Design review of the part built by this model. Coordinates are the model's own, in mm. A direction names the side the tool comes from. Give positions to 0.01 mm unless a question says otherwise; leave off trailing zeros. Loops run counter-clockwise (first coordinate to the right, second up) from the corner with the lowest first, then second, coordinate; pieces in that order, holes last. Notation, with made-up numbers: (54.5, 86) -> (113.5, 86) arc R35 cw to (113.5, 118) -> close; hole circle Ø6 at (1, -16). An arc over 180 degrees is marked (long way). Use CSV: the item, a comma, the result in double quotes. Start each with the question number.
Item 1: Wall thickness on line 1 along Y through (x, z) = (53, 1.6); line 2 along X through (y, z) = (-12, 0.4); line 3 along Y through (x, z) = (-33, 2.55): over which ranges is each line inside the solid? List them lowest first. Write a range as from..to.
Item 2: We need section A-A (x = -23). State the section outline as (y, z) points, plus the area to 3 significant figures.
Item 3: For faces 1 (the face through (1, -49, 1)), 2 (the face through (-60, 1, 1)), list the 3-axis set-ups (+Z, -Z, +X, -X, +Y, -Y) from which the entire face can be reached by the end or side of a thin tool; tool diameter is ignored.
Item 4: Clearance check with a flat-ended pin moving along its axis: pin 1 (6 mm diameter, centred on x = -36, y = -29.5, fed in from -Z). State where the tip first meets the part, or that it passes through.
Item 5: We need section B-B (y = 37). State the section outline as (x, z) points.
Item 6: The part is to be moulded in two halves that separate along X. For faces 3 (the face through (-41, 1, 0)), 4 (the face through (58.196, -67.289, 1.521)), 5 (the face through (-58.289, -67.196, 1.521)), 6 (the face through (50, -62, 2)), say which applies: +X half, -X half, draft (parallel to the pull), parting line (faces both ways), or undercut.
Item 7: We need section C-C (z = 0.6). State the section outline as (x, y) points, plus the area to 3 significant figures.
Autodesk Inventor part; units mm, degrees
ref_plane "YZ Plane" through (0, 0, 0) normal (1, 0, 0) x (0, 1, 0)
ref_plane "XZ Plane" through (0, 0, 0) normal (0, 1, 0) x (-1, 0, 0)
ref_plane "XY Plane" through (0, 0, 0) normal (0, 0, 1) x (1, 0, 0)
sketch "Sketch1" plane through (0, 0, 0) normal (0, 0, 1) x (1, 0, 0)
  line L0 (-60, -69) -> (60, -69)
  line L1 (60, -69) -> (60, 69)
  line L2 (60, 69) -> (-60, 69)
  line L3 (-60, 69) -> (-60, -69)
  line L4 (-60, -69) -> (60, 69) construction
  line L5 (60, -69) -> (-60, 69) construction
  line L6 (40, -49) -> (-40, -49)
  line L7 (-40, -49) -> (-40, 49)
  line L8 (-40, 49) -> (40, 49)
  line L9 (40, 49) -> (40, -49)
  line L10 (40, -49) -> (-40, 49) construction
  line L11 (-40, -49) -> (40, 49) construction
  point P0 (0, 0)
  dimension "d172" = 80
  dimension "d180" = 20
  dimension "d181" = 20
  dimension "d182" = 98
extrude "Plate5" add sketch "Sketch1" along normal blind 3
sketch "Sketch9" plane through (0, 0, 3) normal (0, 0, 1) x (1, 0, 0)
  circle A0 centre (53, -62) radius 3
  line L0 (53, 62) -> (-53, 62) construction
  line L1 (-53, 62) -> (-53, -62) construction
  line L2 (-53, -62) -> (53, -62) construction
  line L3 (53, -62) -> (53, 62) construction
  line L4 (53, 62) -> (-53, -62) construction
  line L5 (-53, 62) -> (53, -62) construction
  circle A1 centre (-53, -62) radius 3
  circle A2 centre (53, 62) radius 3
  circle A3 centre (-53, 62) radius 3
  line L6 (-40, -49) -> (-40, 49)
  line L7 (-40, 49) -> (40, 49)
  line L8 (40, 49) -> (40, -49)
  line L9 (40, -49) -> (-40, -49)
  line L10 (60, -69) -> (-60, -69)
  line L11 (60, 69) -> (60, -69)
  line L12 (-60, 69) -> (60, 69)
  line L13 (-60, -69) -> (-60, 69)
  circle A4 centre (-53, 0) radius 3 construction
  circle A5 centre (53, 0) radius 3 construction
  point P0 (0, 0)
  dimension "d174" = 6
  dimension "d183" = 7
  dimension "d184" = 7
extrude "Cut2" cut sketch "Sketch9" against normal blind 3 contours A0 | A1 | A2 | A3
fillet "Corner Round1" radius 6 4 edges at (60, 69, 1.5) (-60, 69, 1.5) (-60, -69, 1.5) (60, -69, 1.5)
properties part number "ANP 1421 FDS Diam way flange 1" material "Stainless Steel"
Results found:
1,line 1,"-69..-65, -59..59, 65..69"
1,line 2,"-60..-40, 40..60"
1,line 3,"-69..-49, 49..69"
2,outline,"(-69, 0) -> (-49, 0) -> (-49, 3) -> (-69, 3) -> close; (49, 0) -> (69, 0) -> (69, 3) -> (49, 3) -> close"
2,area,"120 mm²"
3,face 1,"+Z, -Z"
3,face 2,"+Z, -Z, -X, +Y, -Y"
4,pin 1,"through"
5,outline,"(-60, 0) -> (-40, 0) -> (-40, 3) -> (-60, 3) -> close; (40, 0) -> (60, 0) -> (60, 3) -> (40, 3) -> close"
6,face 3,"draft"
6,face 4,"+X half"
6,face 5,"-X half"
6,face 6,"undercut"
7,outline,"(-60, -63) arc R6 ccw to (-54, -69) -> (54, -69) arc R6 ccw to (60, -63) -> (60, 63) arc R6 ccw to (54, 69) -> (-54, 69) arc R6 ccw to (-60, 63) -> close; hole circle Ø6 at (-53, -62); hole circle Ø6 at (-53, 62); hole (-40, -49) -> (40, -49) -> (40, 49) -> (-40, 49) -> close; hole circle Ø6 at (53, -62); hole circle Ø6 at (53, 62)"
7,area,"8,580 mm²"
